Model file for the job. Use its own axes, mm. A direction names the side the tool comes from. Round coordinates to 2 decimals unless told otherwise and drop trailing zeros. Loops run counter-clockwise (first coordinate to the right, second up) from the corner with the lowest first, then second, coordinate; pieces in that order, holes last. Notation, with made-up numbers: (30.5, 71) -> (80.5, 71) arc R14 ccw to (80.5, 97) -> close; hole circle Ø11 at (69.5, -1.75). An arc over 180 degrees is marked (long way). Use a Markdown table: item, result.
from build123d import *

# Parameters (mm, degrees)
SKETCH1_R           = 80
BOSS_EXTRUDE1_DEPTH = 15
SKETCH2_R           = 50
BOSS_EXTRUDE2_DEPTH = 75
SKETCH3_R           = 15
CUT_EXTRUDE1_DEPTH  = 91
SKETCH5_R           = 7.5
CUT_EXTRUDE2_DEPTH  = 75
CIRPATTERN1_COUNT   = 4
CUT_EXTRUDE3_DEPTH  = 91


with BuildPart() as part:
    # Sketch1 → Boss-Extrude1 (new body)
    with BuildSketch(Plane(origin=(0, 0, 0), x_dir=(1, 0, 0), z_dir=(0, 1, 0))):
        Circle(SKETCH1_R)
    extrude(amount=BOSS_EXTRUDE1_DEPTH)

    # Sketch2 → Boss-Extrude2 (add)
    with BuildSketch(Plane(origin=(0, 15, 0), x_dir=(1, 0, 0), z_dir=(0, 1, 0))):
        Circle(SKETCH2_R)
    extrude(amount=BOSS_EXTRUDE2_DEPTH)

    # Sketch3 → Cut-Extrude1 (cut, through all)
    with BuildSketch(Plane(origin=(0, 0, 0), x_dir=(1, 0, 0), z_dir=(0, 1, 0))):
        Circle(SKETCH3_R)
    extrude(amount=CUT_EXTRUDE1_DEPTH, mode=Mode.SUBTRACT)

    # Sketch4 → Cut-Revolve1 (revolve, cut)
    with BuildSketch(Plane(origin=(0, 0, 0), x_dir=(0, 0, -1), z_dir=(1, 0, 0))):
        Polygon((-30, 90), (-30, 70), (-50, 15), (-50, 90), align=None)
    revolve(axis=Axis((0, 90, 0), (0, -1, 0)), mode=Mode.SUBTRACT)

    # Sketch5 → Cut-Extrude2 (cut)
    with BuildSketch(Plane.XZ):
        with Locations((0, -65)):
            Circle(SKETCH5_R)
    cut_extrude2 = extrude(amount=-CUT_EXTRUDE2_DEPTH, mode=Mode.SUBTRACT)

    # CirPattern1: Cut-Extrude2 ×4 about axis
    cirpattern1_axis = Axis((0, 0, 0), (0, 1, 0))
    for i in range(1, CIRPATTERN1_COUNT):
        add(cut_extrude2.rotate(cirpattern1_axis, i * 360 / CIRPATTERN1_COUNT), mode=Mode.SUBTRACT)

    # Sketch6 → Cut-Extrude3 (cut, through all)
    with BuildSketch(Plane.XZ):
        Polygon((0, 80), (0, 0), (80, 0), (80, 86.210661468), align=None)
    extrude(amount=-CUT_EXTRUDE3_DEPTH, mode=Mode.SUBTRACT)


solid = part.part
Q1. Band-saw the part on D-D, the plane z = 65. Give the cut face in (x, y), plus the area to 3 significant figures.
Results list:
| item | result |
|---|---|
| outline | (-46.64, 0) -> (-7.5, 0) -> (-7.5, 15) -> (-46.64, 15) -> close |
| area | 587 mm² |
Q2. Band-saw the part on C-C, the plane y = 72.5. Give the cut face in (x, z), plus the area to 3 significant figures.
Results list:
| item | result |
|---|---|
| outline | (0, 15) -> (0, 30) arc R30 ccw (long way) to (30, 0) -> (15, 0) arc R15 cw (long way) to start |
| area | 1,590 mm² |
Q3. Flat gauge pins, fed straight in: pin 1 (5 mm diameter, centred on x = 1, y = 15.5, fed in from -Z); pin 2 (4 mm diameter, centred on x = 75, y = 7, fed in from +Z); pin 3 (3 mm diameter, centred on y = 68, z = 19.5, fed in from -X). Where does each tip first touch, or does it go through?
Results list:
| item | result |
|---|---|
| pin 1 | stops at z = -80 |
| pin 2 | stops at z = 0 |
| pin 3 | stops at x = -25.09 |
Q4. Band-saw the part on A-A, the plane z = -65. Give the cut face in (x, y).
Results list:
| item | result |
|---|---|
| outline | (-46.64, 0) -> (-7.5, 0) -> (-7.5, 15) -> (-46.64, 15) -> close; (7.5, 0) -> (46.64, 0) -> (46.64, 15) -> (7.5, 15) -> close |
Q5. Drill centre lines: L1, parallel to X at y = 7, z = -68; L2, parallel to Y at x = -43.5, z = 52; L3, parallel to Z at x = -10, y = 11.5. Where is each one in solid material? Low to high. Write a range as from..to.
Results list:
| item | result |
|---|---|
| L1 | x = -42.14..-6.87, 6.87..42.14 |
| L2 | y = 0..15 |
| L3 | z = -79.37..-11.18, 11.18..79.37 |
Q6. Pull direction X, two halves, no side cores. Call faces 1 (the face through (-0.976, 7.395, -57.564)), 2 (the face through (0, 7, 76)), 3 (the face through (-21.901, 79.86, -20.502)): released by +X, released by -X, zero draft, split by the parting line, or undercut.
Results list:
| item | result |
|---|---|
| face 1 | undercut |
| face 2 | released by +X |
| face 3 | split by the parting line |
Q7. Band-saw the part on B-B, the plane x = -65. Give the cut face in (y, z).
Results list:
| item | result |
|---|---|
| outline | (0, -46.64) -> (15, -46.64) -> (15, -7.5) -> (0, -7.5) -> close; (0, 7.5) -> (15, 7.5) -> (15, 46.64) -> (0, 46.64) -> close |
Q8. Tool access for faces 4 (the face through (-19, 0, -1)), 5 (the face through (-37, 15, -37)), 6 (the face through (31, 34, 0)): list every direction of +Z, -Z, +X, -X, +Y, -Y with a clear straight run to the whole face (end or side of a thin tool).
Results list:
| item | result |
|---|---|
| face 4 | +Z, -Z, +X, -X, -Y |
| face 5 | +Y |
| face 6 | +Z, +X, +Y, -Y |
